Study the drawing (mm; zero at the part's minimum x, y, z) and answer. Round coordinates to 2 decimals unless told otherwise and drop trailing zeros. Write each loop counter-clockwise with the first axis right and the second up, starting at its lowest first coordinate (ties: lowest second). Pieces come first, ordered by that corner, then holes.
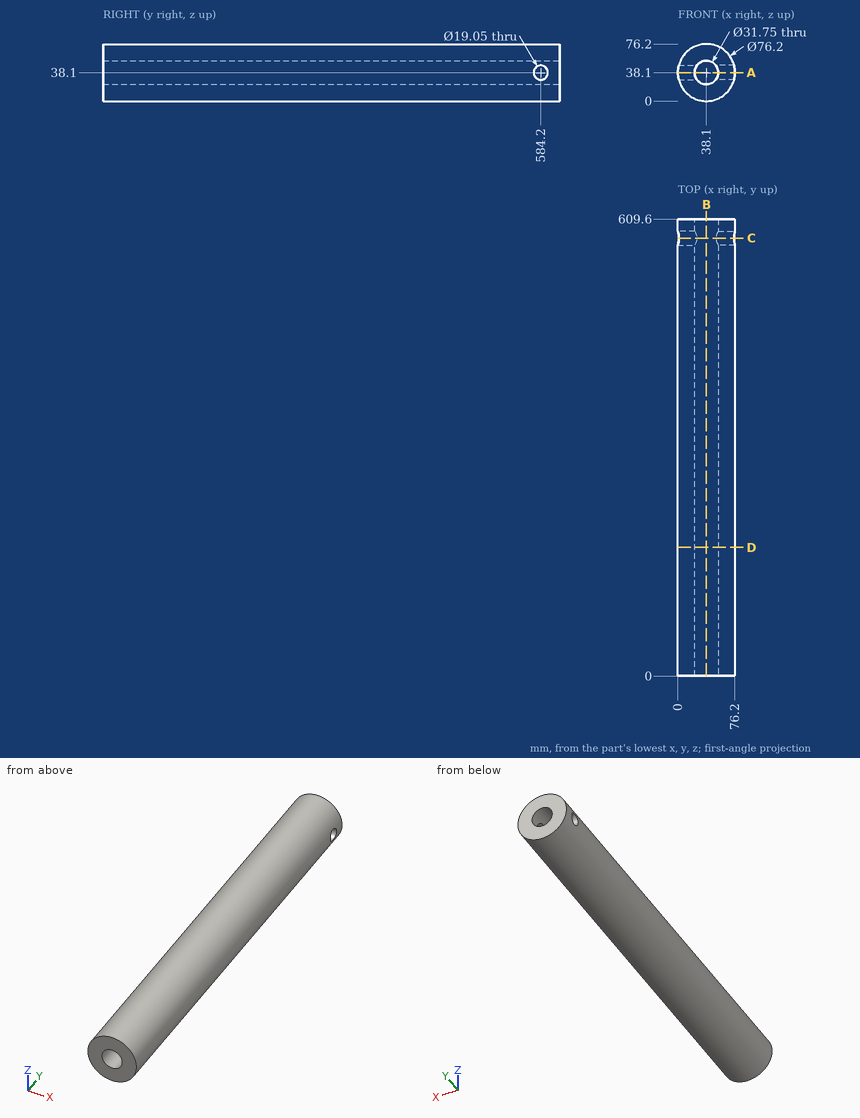
1. Given pin 1 (8 mm diameter, centred on y = 458, z = 27, fed in from +X); pin 2 (1 mm diameter, centred on y = 106.5, z = 49, fed in from -X); pin 3 (12 mm diameter, centred on y = 251.5, z = 45.5, fed in from +X), each flat-ended and moving along its own axis, determine where each tip first touches the part or whether it passes through.
Geometry says:
pin 1: stops at x = 75.53
pin 2: stops at x = 1.45
pin 3: stops at x = 76.17
2. Section D-D on y = 171.5 is taken. Determine the outline of the cut face in (x, z) (3 decimals).
Geometry says:
outline: circle Ø76.2 at (38.1, 38.1); hole circle Ø31.75 at (38.1, 38.1)
3. Straight lines are drawn through the part: line 1 along Z through (x, y) = (39.5, 92); line 2 along Z through (x, y) = (51, 143); line 3 along X through (y, z) = (204.5, 48). For each, find the intervals that lie inside material, in ascending order.
Geometry says:
line 1: z = 0.03 to 22.29, 53.91 to 76.17
line 2: z = 2.25 to 28.85, 47.35 to 73.95
line 3: x = 1.31 to 25.69, 50.51 to 74.89
4. Section B-B on x = 38.1 is taken. Determine the outline of the cut face in (y, z) (3 decimals).
Geometry says:
outline: (0, 0) - (609.6, 0) - (609.6, 22.225) - (0, 22.225) - close; (0, 53.975) - (609.6, 53.975) - (609.6, 76.2) - (0, 76.2) - close
5. Section A-A on z = 38.1 is taken. Determine the outline of the cut face in (x, y) (3 decimals).
Geometry says:
outline: (0, 0) - (22.225, 0) - (22.225, 574.675) - (0, 574.675) - close; (0, 593.725) - (22.225, 593.725) - (22.225, 609.6) - (0, 609.6) - close; (53.975, 0) - (76.2, 0) - (76.2, 574.675) - (53.975, 574.675) - close; (53.975, 593.725) - (76.2, 593.725) - (76.2, 609.6) - (53.975, 609.6) - close
6. Section C-C on y = 584.2 is taken. Determine the outline of the cut face in (x, z) (3 decimals), plus the area to 3 significant figures.
Geometry says:
outline: (1.21, 28.575) arc R38.1 ccw to (74.99, 28.575) - (50.8, 28.575) arc R15.875 cw to (25.4, 28.575) - close; (1.21, 47.625) - (25.4, 47.625) arc R15.875 cw to (50.8, 47.625) - (74.99, 47.625) arc R38.1 ccw to start
area: 2,900 mm2
